Verification items for the finished model (mm, model axes). A direction names the side the tool comes from. Round coordinates to 2 decimals unless told otherwise and drop trailing zeros. Loops run counter-clockwise (first coordinate to the right, second up) from the corner with the lowest first, then second, coordinate; pieces in that order, holes last.
from build123d import *

# Parameters (mm, degrees)
SKETCH1_R           = 11.1125
SKETCH1_R_2         = 2.413
BOSS_EXTRUDE1_DEPTH = 5.842


with BuildPart() as part:
    # Sketch1 → Boss-Extrude1 (new body)
    with BuildSketch(Plane(origin=(0, 0, 0), x_dir=(1, 0, 0), z_dir=(0, 1, 0))):
        Polygon((25.4, -21.1058), (19.05, -21.1058), (19.05, -26.9478), (6.35, -26.9478), (6.35, -21.1058), (1.778, -21.1058), (1.778, -17.9308), (3.048, -17.9308), (3.048, -14.7558), (1.778, -14.7558), (1.778, -14.2478), (-1.778, -14.2478), (-1.778, -14.7558), (-3.048, -14.7558), (-3.048, -17.9308), (-1.778, -17.9308), (-1.778, -21.1058), (-6.35, -21.1058), (-6.35, -26.9478), (-19.05, -26.9478), (-19.05, -21.1058), (-25.4, -21.1058), (-25.4, 21.1058), (-19.05, 21.1058), (-19.05, 26.9478), (-6.35, 26.9478), (-6.35, 21.1058), (-1.778, 21.1058), (-1.778, 17.9308), (-3.048, 17.9308), (-3.048, 14.7558), (-1.778, 14.7558), (-1.778, 14.2478), (1.778, 14.2478), (1.778, 14.7558), (3.048, 14.7558), (3.048, 17.9308), (1.778, 17.9308), (1.778, 21.1058), (6.35, 21.1058), (6.35, 26.9478), (19.05, 26.9478), (19.05, 21.1058), (25.4, 21.1058), align=None)
        with Locations(Location((0, 0, 0), (0, 0, 270))):
            Circle(SKETCH1_R, mode=Mode.SUBTRACT)
        with Locations(Location((-17.960512242, 17.960512242, 0), (0, 0, 270))):
            Circle(SKETCH1_R_2, mode=Mode.SUBTRACT)
        with Locations(Location((17.960512242, 17.960512242, 0), (0, 0, 270))):
            Circle(SKETCH1_R_2, mode=Mode.SUBTRACT)
        with Locations(Location((17.960512242, -17.960512242, 0), (0, 0, 270))):
            Circle(SKETCH1_R_2, mode=Mode.SUBTRACT)
        with Locations(Location((-17.960512242, -17.960512242, 0), (0, 0, 270))):
            Circle(SKETCH1_R_2, mode=Mode.SUBTRACT)
    extrude(amount=BOSS_EXTRUDE1_DEPTH)


solid = part.part
1. Scan lines: L1, parallel to X at y = 4, z = 0; L2, parallel to X at y = 2.45, z = -20.5; L3, parallel to Z at x = -17, y = 2.65. Record each from-to range of solid material in increasing order.
2. Gauge pin test, flat ends, axial feed: P1, Ø1.1, axis at x = 0, y = 3, coming from the +Z side; P2, Ø6, axis at x = 3, z = 9.5, coming from the -Y side; P3, Ø1.5, axis at x = 4, y = 2.5, coming from the -Z side; P4, Ø1.8, axis at x = 0.5, y = 2, coming from the -Z side. Record the tip position at first contact, or that the pin passes through.
3. Tool access check on faces 1 (the face through (2, 3, -17.931)), 2 (the face through (19.05, 3, 24)), 3 (the face through (-19.05, 3, -24)). Record the directions out of +Z, -Z, +X, -X, +Y, -Y that give a thin tool (end or side, any length) a straight path to the whole face; none if there is none.
4. Section check C-C (y = 1.45). Give the number of separate pieces and of enclosed holes in the cut face, then the cut area to 3 significant figures.
5. Section check A-A (x = 0). Enter the section's corners in (y, z).
6. Section check B-B (z = 0). Enter the section's corners in (x, y).
7. Release check for a two-part mould opening along Z. For faces 4 (the face through (0, 3, 14.248)), 5 (the face through (9.37, 2.88, 5.974)), 6 (the face through (12, 5.842, 0)) record: released by +Z, released by -Z, zero draft, split by the parting line, or undercut.
Taken from the geometry:
1. L1: x = -25.4 to -11.11, 11.11 to 25.4
1. L2: x = -25.4 to -1.78, 1.78 to 25.4
1. L3: z = -26.95 to -20.17, -15.75 to 15.75, 20.17 to 26.95
2. P1: stops at z = 14.25
2. P2: stops at y = 0
2. P3: stops at z = -21.11
2. P4: stops at z = -14.25
3. face 1: +Y, -Y
3. face 2: +Z, +X, +Y, -Y
3. face 3: -Z, -X, +Y, -Y
4. separate pieces: 1
4. enclosed holes: 5
4. area: 1,920 mm2
5. outline: (0, -14.25) - (5.84, -14.25) - (5.84, -11.11) - (0, -11.11) - close; (0, 11.11) - (5.84, 11.11) - (5.84, 14.25) - (0, 14.25) - close
6. outline: (-25.4, 0) - (-11.11, 0) - (-11.11, 5.84) - (-25.4, 5.84) - close; (11.11, 0) - (25.4, 0) - (25.4, 5.84) - (11.11, 5.84) - close
7. face 4: released by +Z
7. face 5: undercut
7. face 6: zero draft
